from build123d import *

# Parameters (mm, degrees)
BOSS_EXTRU_1_DEPTH                                  = 15
CBORE_FOR_M6_HEX_SOCKET_HEAD_CAP_SCREW1_D           = 6.6
CBORE_FOR_M6_HEX_SOCKET_HEAD_CAP_SCREW1_CBORE_D     = 11
CBORE_FOR_M6_HEX_SOCKET_HEAD_CAP_SCREW1_CBORE_DEPTH = 6.4
CBORE_FOR_M8_HEX_SOCKET_HEAD_CAP_SCREW1_D           = 9
CBORE_FOR_M8_HEX_SOCKET_HEAD_CAP_SCREW1_CBORE_D     = 15
CBORE_FOR_M8_HEX_SOCKET_HEAD_CAP_SCREW1_CBORE_DEPTH = 8.6
TAP_DRILL_FOR_M6_TAP1_D                             = 5
TAP_DRILL_FOR_M3_TAP1_D                             = 2.5
CUT_EXTRUDE1_DEPTH                                  = 16
FILLET3_R                                           = 10
FILLET4_R                                           = 3
CHAMFER1_SIZE                                       = 0.5


with BuildPart() as part:
    # Esquisse1 → Boss.-Extru.1 (new body)
    with BuildSketch(Plane.XY):
        Polygon((3, 169), (3, 17.5), (20.5, 0), (68.5, 0), (118.5, 0), (118.5, 190), (68.5, 190), (24, 190), align=None)
    extrude(amount=BOSS_EXTRU_1_DEPTH)

    # CBORE for M6 Hex Socket Head Cap Screw1 (through all)
    with Locations(Plane.XY.offset(15)):
        with Locations((83, 30), (107, 140), (107, 30), (83, 140)):
            CounterBoreHole(CBORE_FOR_M6_HEX_SOCKET_HEAD_CAP_SCREW1_D / 2, CBORE_FOR_M6_HEX_SOCKET_HEAD_CAP_SCREW1_CBORE_D / 2, CBORE_FOR_M6_HEX_SOCKET_HEAD_CAP_SCREW1_CBORE_DEPTH)

    # CBORE for M8 Hex Socket Head Cap Screw1 (through all)
    with Locations(Plane.XY.offset(15)):
        with Locations((71, 107.5), (71, 62.5), (14, 62.5), (14, 107.5)):
            CounterBoreHole(CBORE_FOR_M8_HEX_SOCKET_HEAD_CAP_SCREW1_D / 2, CBORE_FOR_M8_HEX_SOCKET_HEAD_CAP_SCREW1_CBORE_D / 2, CBORE_FOR_M8_HEX_SOCKET_HEAD_CAP_SCREW1_CBORE_DEPTH)

    # Tap Drill for M6 Tap1 (through all)
    with Locations(Plane.XY.offset(15)):
        with Locations((92.5, 7.5)):
            Hole(TAP_DRILL_FOR_M6_TAP1_D / 2)

    # Tap Drill for M3 Tap1 (through all)
    with Locations(Plane(origin=(0, 0, 0), x_dir=(-1, 0, 0), z_dir=(0, 0, -1))):
        with Locations((-24.2, 35), (-13.8, 35), (-24.2, 135), (-13.8, 135)):
            Hole(TAP_DRILL_FOR_M3_TAP1_D / 2)

    # Sketch17 → Cut-Extrude1 (cut, through all)
    with BuildSketch(Plane.XY.offset(15)):
        with BuildLine():
            Line((12, 118.8), (-6, 118.8))
            ThreePointArc((-6, 118.8), (-12.2, 125), (-6, 131.2))
            Line((-6, 131.2), (12, 131.2))
            ThreePointArc((12, 131.2), (18.2, 125), (12, 118.8))
        make_face()
        with BuildLine():
            Line((15.5, 38.8), (-2.5, 38.8))
            ThreePointArc((-2.5, 38.8), (-8.7, 45), (-2.5, 51.2))
            Line((-2.5, 51.2), (15.5, 51.2))
            ThreePointArc((15.5, 51.2), (21.7, 45), (15.5, 38.8))
        make_face()
    extrude(amount=-CUT_EXTRUDE1_DEPTH, mode=Mode.SUBTRACT)

    # Fillet3
    fillet3_edges = [part.edges().sort_by_distance(p)[0] for p in [
        (20.5, 0, 7.5),
        (3, 17.5, 7.5),
        (3, 169, 7.5),
        (24, 190, 7.5),
    ]]
    fillet(fillet3_edges, radius=FILLET3_R)

    # Fillet4
    fillet4_edges = [part.edges().sort_by_distance(p)[0] for p in [
        (3, 118.8, 7.5),
        (3, 131.2, 7.5),
        (3, 38.8, 7.5),
        (3, 51.2, 7.5),
    ]]
    fillet(fillet4_edges, radius=FILLET4_R)

    # Chamfer1
    chamfer1_edges = [part.edges().sort_by_distance(p)[0] for p in [
        (22.95, 35, 15),
        (10.75, 38.8, 15),
        (9, 118.8, 15),
        (9, 131.2, 15),
        (18.2, 125, 15),
        (10.75, 51.2, 15),
        (21.7, 45, 15),
        (3, 149.528932188, 15),
        (13.5, 179.5, 15),
        (11.75, 8.75, 15),
        (71.571067812, 0, 15),
        (20.8153013, 0.761204675, 15),
        (24.3153013, 189.238795325, 15),
        (3.761204675, 17.8153013, 15),
        (3.761204675, 168.6846987, 15),
        (3, 85, 15),
        (3, 28.721067812, 15),
        (3.878679656, 37.921320344, 15),
        (3.878679656, 52.078679656, 15),
        (3.878679656, 132.078679656, 15),
        (3.878679656, 117.921320344, 15),
        (118.5, 95, 15),
        (77.5, 140, 15),
        (101.5, 30, 15),
        (101.5, 140, 15),
        (73.321067812, 190, 15),
        (77.5, 30, 15),
        (6.5, 107.5, 15),
        (6.5, 62.5, 15),
        (63.5, 62.5, 15),
        (63.5, 107.5, 15),
        (12.55, 135, 15),
        (22.95, 135, 15),
        (12.55, 35, 15),
    ]]
    chamfer(chamfer1_edges, length=CHAMFER1_SIZE)


solid = part.part
Build history of the part. All positions in model axes, mm. A direction names the side the tool comes from. Coordinates: 2 decimals unless noted, no trailing zeros. Order: outer loops, then holes, each group sorted by start corner. A loop starts at its lowest first (then second) coordinate and runs counter-clockwise, first axis right, second up. Notation, with made-up numbers: (31.5, 46) -> (78.5, 46) arc R16 ccw to (78.5, 68) -> close; hole circle Ø1 at (65, -2.5). An arc over 180 degrees is marked (long way). One line per item, written item: value.
(1) Slice it at A-A, the plane x = 71. List the corners of the cut face in (y, z).
Checked values:
outline: (0, 0) -> (58, 0) -> (58, 6.4) -> (55, 6.4) -> (55, 14.5) -> (54.5, 15) -> (0.5, 15) -> (0, 14.5) -> close; (67, 0) -> (103, 0) -> (103, 6.4) -> (100, 6.4) -> (100, 14.5) -> (99.5, 15) -> (70.5, 15) -> (70, 14.5) -> (70, 6.4) -> (67, 6.4) -> close; (112, 0) -> (190, 0) -> (190, 14.5) -> (189.5, 15) -> (115.5, 15) -> (115, 14.5) -> (115, 6.4) -> (112, 6.4) -> close
(2) Tool access for faces 1 (the flat face through (87, 30, 8.6)), 2 (the flat face through (11, 38.8, 7)), 3 (the flat face through (74, 190, 7)): list every direction of +Z, -Z, +X, -X, +Y, -Y with a clear straight run to the whole face (end or side of a thin tool).
Checked values:
face 1: +Z
face 2: +Z, -Z, -X
face 3: +Z, -Z, +X, -X, +Y
(3) Probe line 1 (Y direction, x = 70.5, z = 12.75); line 2 (Y direction, x = 107, z = 4.5); line 3 (X direction, y = 112, z = 12.75). List the from-to ranges inside material, lowest first. Write a range as [from, to].
Checked values:
line 1: [0, 55.02], [69.98, 100.02], [114.98, 190]
line 2: [0, 26.7], [33.3, 136.7], [143.3, 190]
line 3: [3, 8], [20, 65], [77, 118.5]
(4) Slice it at D-D, the plane y = 7.5. List the corners of the cut face in (x, z), plus the area to 3 significant figures.
Checked values:
outline: (13, 0) -> (90, 0) -> (90, 15) -> (13.71, 15) -> (13, 14.5) -> close; (95, 0) -> (118.5, 0) -> (118.5, 14.5) -> (118, 15) -> (95, 15) -> close
area: 1,510 mm2
(5) Slice it at C-C, the plane x = 92.5. List the corners of the cut face in (y, z), plus the area to 3 significant figures.
Checked values:
outline: (0, 0) -> (5, 0) -> (5, 15) -> (0.5, 15) -> (0, 14.5) -> close; (10, 0) -> (190, 0) -> (190, 14.5) -> (189.5, 15) -> (10, 15) -> close
area: 2,770 mm2
(6) Slice it at B-B, the plane y = 30. List the corners of the cut face in (x, z).
Checked values:
outline: (3, 0) -> (79.7, 0) -> (79.7, 8.6) -> (77.5, 8.6) -> (77.5, 14.5) -> (77, 15) -> (3.5, 15) -> (3, 14.5) -> close; (86.3, 0) -> (103.7, 0) -> (103.7, 8.6) -> (101.5, 8.6) -> (101.5, 14.5) -> (101, 15) -> (89, 15) -> (88.5, 14.5) -> (88.5, 8.6) -> (86.3, 8.6) -> close; (110.3, 0) -> (118.5, 0) -> (118.5, 14.5) -> (118, 15) -> (113, 15) -> (112.5, 14.5) -> (112.5, 8.6) -> (110.3, 8.6) -> close
(7) Drop flat-ended pins along their axis: pin 1 Ø17.5 at (x, y) = (83, 30) entering from -Z; pin 2 Ø7.5 at (x, y) = (72, 64) entering from +Z; pin 3 Ø5.5 at (x, y) = (83, 30) entering from -Z; pin 4 Ø6.5 at (x, z) = (8, 6) entering from -Y. Give the stop position or say it passes through.
Checked values:
pin 1: z = 0
pin 2: z = 6.4
pin 3: through
pin 4: y = 9.25
